Build history of the part. All positions in model axes, mm. Face numbers are marked on the shaded views. A direction names the side the tool comes from. Give positions to 0.01 mm unless a question says otherwise; leave off trailing zeros. Loops run counter-clockwise (first coordinate to the right, second up) from the corner with the lowest first, then second, coordinate; pieces in that order, holes last. Notation, with made-up numbers: M 10,59 L 57,59 A32 ccw 57,91 Z; hole C 45,52.5 d7. An arc over 180 degrees is marked long. Answer as a JSON object with one key per item and string values. Group by question number.
1. Slice it at C-C (y = -6). List the corners of the cut face in (x, z).
2. Drill centre lines: line 1 along X through (y, z) = (-10.75, -37.5); line 2 along Z through (x, y) = (11.43, -9.75); line 3 along X through (y, z) = (-5.5, -64). Where is each one in solid material? Low to high. Write a range as [from, to].
3. Slice it at D-D (x = 45). List the corners of the cut face in (y, z), then the cut area to 3 significant figures.
4. 3-axis set-ups, long thin cutter, end or side, ignore diameter. For the marked faces 1, 2 and 3: which of +Z, -Z, +X, -X, +Y, -Y reach the whole face in a straight line?
5. Slice it at B-B (x = 14). List the corners of the cut face in (y, z).
6. Drop flat-ended pins along their axis: pin 1 Ø12.5 at (x, z) = (11.43, -11.11) entering from -Y; pin 2 Ø5 at (x, z) = (123.19, -11.11) entering from +Y; pin 3 Ø19 at (x, z) = (123, -37) entering from +Y; pin 4 Ø1.9 at (y, z) = (2, -37) entering from -X. Give the stop position or say it passes through.
7. Slice it at A-A (z = -18). List the corners of the cut face in (x, y), then the cut area to 3 significant figures.
from build123d import *

# Parameters (mm, degrees)
SKETCH1_R           = 3.96875
BOSS_EXTRUDE1_DEPTH = 12.7
SKETCH3_W           = 58.42
SKETCH3_H           = 76.2
BOSS_EXTRUDE2_DEPTH = 3.81
SKETCH4_W           = 47.625
SKETCH4_H           = 76.2
CUT_EXTRUDE1_DEPTH  = 3.9624


with BuildPart() as part:
    # Sketch1 → Boss-Extrude1 (new body)
    with BuildSketch(Plane(origin=(0, 0, 0), x_dir=(1, 0, 0), z_dir=(0, 1, 0))):
        with BuildLine():
            Line((12.7, 76.2), (121.92, 76.2))
            ThreePointArc((121.92, 76.2), (130.900256121, 72.480256121), (134.62, 63.5))
            Line((134.62, 63.5), (134.62, 12.7))
            ThreePointArc((134.62, 12.7), (130.900256121, 3.719743879), (121.92, 0))
            Line((121.92, 0), (12.7, 0))
            ThreePointArc((12.7, 0), (3.719743879, 3.719743879), (0, 12.7))
            Line((0, 12.7), (0, 63.5))
            ThreePointArc((0, 63.5), (3.719743879, 72.480256121), (12.7, 76.2))
        make_face()
        with Locations((11.43, 65.0875)):
            Circle(SKETCH1_R, mode=Mode.SUBTRACT)
        with Locations((123.19, 65.0875)):
            Circle(SKETCH1_R, mode=Mode.SUBTRACT)
        with Locations((123.19, 11.1125)):
            Circle(SKETCH1_R, mode=Mode.SUBTRACT)
        with Locations((11.43, 11.1125)):
            Circle(SKETCH1_R, mode=Mode.SUBTRACT)
    extrude(amount=-BOSS_EXTRUDE1_DEPTH)

    # Sketch3 → Boss-Extrude2 (add)
    with BuildSketch(Plane(origin=(0, 0, 0), x_dir=(1, 0, 0), z_dir=(0, 1, 0))):
        with Locations((67.31, 38.1)):
            Rectangle(SKETCH3_W, SKETCH3_H)
    extrude(amount=BOSS_EXTRUDE2_DEPTH)

    # Sketch4 → Cut-Extrude1 (cut)
    with BuildSketch(Plane.XZ.offset(12.7)):
        with Locations((67.31, -38.1)):
            Rectangle(SKETCH4_W, SKETCH4_H)
    extrude(amount=-CUT_EXTRUDE1_DEPTH, mode=Mode.SUBTRACT)


solid = part.part
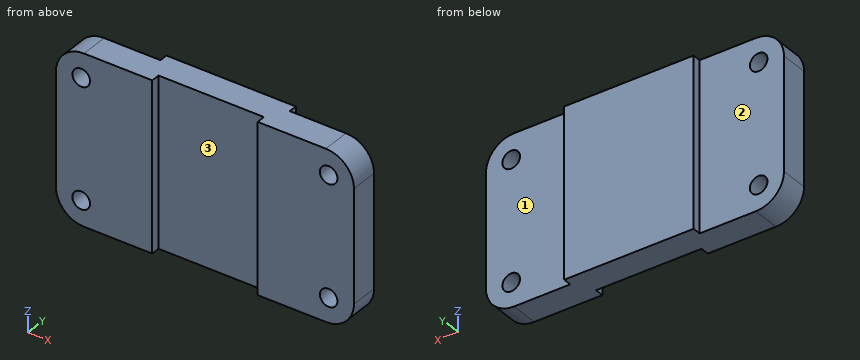
Established:
{
 "1": {"outline": "M 0,-63.5 A12.7 ccw 12.7,-76.2 L 121.92,-76.2 A12.7 ccw 134.62,-63.5 L 134.62,-12.7 A12.7 ccw 121.92,0 L 12.7,0 A12.7 ccw 0,-12.7 Z; hole C 11.43,-65.09 d7.94; hole C 11.43,-11.11 d7.94; hole C 123.19,-65.09 d7.94; hole C 123.19,-11.11 d7.94"},
 "2": {"line 1": "x = [0, 43.5], [91.12, 134.62]", "line 2": "z = [-76.14, -69.06], [-61.12, -15.08], [-7.14, -0.06]", "line 3": "x = [0.01, 7.61], [15.25, 119.37], [127.01, 134.61]"},
 "3": {"outline": "M -8.74,-76.2 L 3.81,-76.2 L 3.81,0 L -8.74,0 Z", "area": "956 mm^2"},
 "4": {"face 1": "+Z, -Z, +X, +Y", "face 2": "+Z, -Z, -X, +Y", "face 3": "+Z, -Z, -Y"},
 "5": {"outline": "M -12.7,-76.2 L 0,-76.2 L 0,-68.11 L -12.7,-68.11 Z; M -12.7,-62.06 L 0,-62.06 L 0,-14.14 L -12.7,-14.14 Z; M -12.7,-8.09 L 0,-8.09 L 0,0 L -12.7,0 Z"},
 "6": {"pin 1": "stops at y = -12.7", "pin 2": "passes through", "pin 3": "stops at y = 0", "pin 4": "stops at x = 38.1"},
 "7": {"outline": "M 0,-12.7 L 43.5,-12.7 L 43.5,-8.74 L 91.12,-8.74 L 91.12,-12.7 L 134.62,-12.7 L 134.62,0 L 96.52,0 L 96.52,3.81 L 38.1,3.81 L 38.1,0 L 0,0 Z", "area": "1,740 mm^2"}
}
